Autodesk Inventor part; units mm, degrees
ref_plane "工作平面2" through (20, 40, 0) normal (-0.8017837, -0.5345225, -0.2672612) x (0.3162278, 0, -0.9486833)
ref_plane "YZ Plane" through (0, 0, 0) normal (1, 0, 0) x (0, 1, 0)
ref_plane "XZ Plane" through (0, 0, 0) normal (0, 1, 0) x (-1, 0, 0)
sketch "草圖1" plane through (0, 0, 0) normal (0, 1, 0) x (-1, 0, 0)
  line L0 (0, 0) -> (-60, 0)
  line L1 (-60, 0) -> (-60, -40)
  line L2 (-60, -40) -> (0, -40)
  line L3 (0, -40) -> (0, 0)
  dimension "d0" = 60
  dimension "d1" = 40
extrude "擠出1" add sketch "草圖1" along normal blind 40
sketch "草圖2" plane through (60, 0, 0) normal (1, 0, 0) x (0, 0, -1)
  line L0 (0, 40) -> (30, 40)
  line L1 (30, 40) -> (30, 10)
  line L2 (30, 10) -> (0, 10)
  line L3 (0, 10) -> (0, 40)
  line L4 (40, 0) -> (40, 40)
  line L5 (0, 0) -> (40, 0)
  dimension "d4" = 10
  dimension "d5" = 10
extrude "擠出2" cut sketch "草圖2" against normal blind 10
sketch "草圖6" plane through (0, 40, 0) normal (0, 1, 0) x (1, 0, 0)
  line L0 (0, 0) -> (60, 0)
  line L1 (60, 30) -> (60, 0)
  line L2 (0, 40) -> (0, 0)
  line L3 (50, 30) -> (60, 30)
  point P0 (20, 0)
  point P1 (30, 30)
  dimension "d12" = 30
  dimension "d13" = 20
  dimension "d14" = 0
sketch "草圖7" plane through (0, 0, 0) normal (0, 0, 1) x (1, 0, 0)
  line L0 (60, 0) -> (60, 10)
  line L1 (60, 10) -> (50, 10)
  point P0 (0, 0)
  point P1 (40, 10)
  dimension "d15" = 20
  dimension "d16" = 0
ref_plane "工作平面2" through (20, 40, 0) normal (-0.8017837, -0.5345225, -0.2672612) x (0.3162278, 0, -0.9486833)
sketch "草圖8" plane through (20, 40, 0) normal (-0.8017837, -0.5345225, -0.2672612) x (0.3162278, 0, -0.9486833)
  line L0 (-6.3246, -10.1419) -> (9.4868, 15.2128)
  line L1 (-1.8957, -3.0399) -> (37.7838, -3.0399)
  line L2 (37.7838, -3.0399) -> (37.7838, 41.2626)
  line L3 (37.7838, 41.2626) -> (-1.8957, 41.2626)
  line L4 (-1.8957, 41.2626) -> (-1.8957, -3.0399)
  point P0 (-6.3246, 23.6643)
extrude "擠出3" cut sketch "草圖8" against normal blind 50
sketch "草圖9" plane through (0, 40, 0) normal (0, 1, 0) x (1, 0, 0)
  line L0 (60, 30) -> (50, 30)
  line L1 (60, 40) -> (0, 40)
  line L2 (60, 30) -> (0, 30)
  line L3 (0, 30) -> (0, 40)
  line L4 (0, 40) -> (60, 40)
  line L5 (60, 40) -> (60, 30)
  point P0 (0, 0)
extrude "擠出4" add sketch "草圖9" against normal up to next
sketch "草圖10" plane through (60, 0, -40) normal (1, 0, 0) x (0, 0, -1)
  line L0 (-10, 40) -> (0, 40)
  line L1 (0, 40) -> (-10, 40)
  line L2 (-10, 40) -> (-10, 0)
  line L3 (-10, 0) -> (0, 0)
  line L4 (0, 0) -> (0, 40)
  line L5 (-40, 0) -> (-40, 40)
  line L6 (0, 0) -> (-40, 0)
  line L7 (-40, 0) -> (-40, 10)
  line L8 (-40, 10) -> (0, 10)
  line L9 (0, 10) -> (0, 0)
  dimension "d21" = 0
  dimension "d22" = 10
  dimension "d23" = 10
extrude "擠出5" add sketch "草圖10" against normal up to next
delete faces "刪除面1" heal yes whole lump no faces at (50, 30, -29.8851) (49.8276, 20.2573, -29.8851)
properties part number "49 (73500.000 mm^3)"
Design review of the part built by this model. Coordinates are the model's own, in mm. A direction names the side the tool comes from. Give positions to 0.01 mm unless a question says otherwise; leave off trailing zeros. Write each loop counter-clockwise with the first axis right and the second up, starting at its lowest first coordinate (ties: lowest second). Pieces come first, ordered by that corner, then holes. Notation, with made-up numbers: M 67.25,39.5 L 96.25,39.5 A17 ccw 96.25,60.5 Z; hole C -3.5,-31.5 d2. An arc over 180 degrees is marked long. Answer as a JSON object with one key per item and string values. Group by question number.
1) We need section C-C (x = 24). Give the boundary of the cut face in (y, z), and give its area (3 significant figures).
2) We need section B-B (z = -16). Give the boundary of the cut face in (x, y).
3) We need section A-A (x = 52). Give the boundary of the cut face in (y, z).
4) Clearance check with flat-ended pins moving along their axes: pin 1 Ø6 at (x, z) = (53.5, -12) entering from +Y; pin 2 Ø4 at (y, z) = (15.5, -16.5) entering from +X. State where each tip first meets the part, or that it passes through.
5) For line 1 along Z through (x, y) = (50, 25); line 2 along Y through (x, z) = (49, -25); line 3 along Y through (x, z) = (42, -26), list the stretches that pass through material, from the lowest coordinate up.
6) Tool access review of faces 1 (the face through (30, 20, -40)), 2 (the face through (49, 29, -30)): name each direction out of +Z, -Z, +X, -X, +Y, -Y from which nothing blocks a thin tool from reaching the whole face with its end or side.
Answer key:
{
 "1": {"outline": "M 0,-40 L 40,-40 L 40,-12.01 L 34,0 L 0,0 Z", "area": "1,560 mm²"},
 "2": {"outline": "M 0,0 L 60,0 L 60,10 L 45.33,10 L 25.33,40 L 0,40 Z"},
 "3": {"outline": "M 0,-40 L 40,-40 L 40,-30 L 10,-30 L 10,0 L 0,0 Z"},
 "4": {"pin 1": "stops at y = 10", "pin 2": "stops at x = 43.32"},
 "5": {"line 1": "z = -40 to -30", "line 2": "y = 0 to 10", "line 3": "y = 0 to 20"},
 "6": {"face 1": "-Z, +X, -X, +Y, -Y", "face 2": "+Z, +X, +Y"}
}
